Verification items for the finished model (mm, model axes). A direction names the side the tool comes from. Round coordinates to 2 decimals unless told otherwise and drop trailing zeros. Loops run counter-clockwise (first coordinate to the right, second up) from the corner with the lowest first, then second, coordinate; pieces in that order, holes last. Notation, with made-up numbers: M 56.25,-8.75 L 70.25,-8.75 A10 cw 70.25,8.25 Z; hole C 27,20 d9. An arc over 180 degrees is marked long. One line per item, written item: value.
Autodesk Inventor part; units mm, degrees
ref_plane "YZ Plane" through (0, 0, 0) normal (1, 0, 0) x (0, 1, 0)
ref_plane "XZ Plane" through (0, 0, 0) normal (0, 1, 0) x (-1, 0, 0)
ref_plane "XY Plane" through (0, 0, 0) normal (0, 0, 1) x (1, 0, 0)
sketch "Boceto1" plane through (0, 0, 0) normal (0, 0, 1) x (1, 0, 0)
  line L0 (0, 132.9544) -> (0, -187.2356) construction
  line L1 (-210.4029, 0) -> (220.8608, 0) construction
  line L2 (0, 47.5) -> (-20.5, 47.5)
  line L3 (0, -47.5) -> (-21.5, -47.5)
  line L4 (-21.5, -47.5) -> (-21.5, 65.7423) construction
  line L5 (-20.5, 47.5) -> (-21.5, 17.5)
  line L6 (-21.5, -47.5) -> (-21.5, 17.5)
  line L7 (0, 47.5) -> (0, -47.5)
  point P0 (0, 0)
  point P1 (-10.75, -47.5)
  point P2 (-10.25, 47.5)
  dimension "d0" = 20.5
  dimension "d1" = 21.5
  dimension "d2" = 95
  dimension "d3" = 30
revolve "Revolución1" add sketch "Boceto1" angle 360 about axis through (0, 132.9544, 0) along (0, -1, 0)
sketch "Boceto2" plane through (0, 47.5, 0) normal (0, 1, 0) x (1, 0, 0)
  circle A0 centre (0, 0) radius 17.5
  dimension "d5" = 35
extrude "Extrusión1" cut sketch "Boceto2" against normal blind 150
sketch "Boceto3" plane through (0, -47.5, 0) normal (0, -1, 0) x (1, 0, 0)
  circle A0 centre (0, 0) radius 18.5
  dimension "d8" = 37
extrude "Extrusión2" cut sketch "Boceto3" against normal blind 65
(1) Sectioned sample at D-D on y = 23. Enter the section's corners in (x, z), and give its area (3 significant figures).
Completed:
outline: C 0,0 d42.63; hole C 0,0 d35
area: 465 mm^2
(2) Tool access check on faces 1 (the face through (-15.1, 47.5, -9.2)), 2 (the face through (-11, 17.5, -14)). Record the directions out of +Z, -Z, +X, -X, +Y, -Y that give a thin tool (end or side, any length) a straight path to the whole face; none if there is none.
Completed:
face 1: +Z, -Z, +X, -X, +Y
face 2: -Y
(3) Sectioned sample at A-A on x = 0. Enter the section's corners in (y, z), and give its area (3 significant figures).
Completed:
outline: M -47.5,-21.5 L 17.5,-21.5 L 47.5,-20.5 L 47.5,-17.5 L 17.5,-17.5 L 17.5,-18.5 L -47.5,-18.5 Z; M -47.5,18.5 L 17.5,18.5 L 17.5,17.5 L 47.5,17.5 L 47.5,20.5 L 17.5,21.5 L -47.5,21.5 Z
area: 600 mm^2
(4) Sectioned sample at C-C on y = -3.5. Enter the section's corners in (x, z).
Completed:
outline: C 0,0 d43; hole C 0,0 d37
(5) Mould release check, pull along Z, two halves, no side actions. Record for faces 3 (the face through (4.55, 32.29, 20.51)), 4 (the face through (-13.887, 32.71, 10.648)), 5 (the face through (-6, -47.5, -18)): +Z half, -Z half, draft (parallel to the pull), parting line (faces both ways), or undercut.
Completed:
face 3: parting line
face 4: undercut
face 5: draft
(6) Thickness scan on L1, parallel to Z at x = 0, y = -9; L2, parallel to X at y = -12, z = -4; L3, parallel to Z at x = -10, y = -33.5. Record the ranges inside material, lowest first. Write a range as from..to.
Completed:
L1: z = -21.5..-18.5, 18.5..21.5
L2: x = -21.12..-18.06, 18.06..21.12
L3: z = -19.03..-15.56, 15.56..19.03
(7) Depth check by flat-ended pin: pin 1 Ø4 at (y, z) = (-6.5, 17) entering from +X; pin 2 Ø5 at (y, z) = (-11, -5) entering from -X; pin 3 Ø12 at (x, y) = (0.5, 21) entering from +Z. Enter the tip coordinate at first touch or a pass-through.
Completed:
pin 1: stops at x = 15.4
pin 2: stops at x = -21.35
pin 3: stops at z = 21.5
(8) Sectioned sample at B-B on z = 0. Enter the section's corners in (x, y), and give its area (3 significant figures).
Completed:
outline: M -21.5,-47.5 L -18.5,-47.5 L -18.5,17.5 L -17.5,17.5 L -17.5,47.5 L -20.5,47.5 L -21.5,17.5 Z; M 17.5,17.5 L 18.5,17.5 L 18.5,-47.5 L 21.5,-47.5 L 21.5,17.5 L 20.5,47.5 L 17.5,47.5 Z
area: 600 mm^2
